```python
from build123d import *

# Parameters (mm, degrees)
SKETCH_1_R      = 40.9
SKETCH_1_R_2    = 1.55
EXTRUDE_1_DEPTH = 30


with BuildPart() as part:
    # 草图1 → 凸台-拉伸1 (new body)
    with BuildSketch(Plane(origin=(0, 0, 0), x_dir=(1, 0, 0), z_dir=(0, 1, 0))):
        with BuildLine():
            ThreePointArc((2.968149583, 44.335990888), (0, 46.9), (-2.968149583, 44.335990888))
            ThreePointArc((-2.968149583, 44.335990888), (-3.557987573, 43.187596963), (-4.726563367, 42.638827361))
            ThreePointArc((-4.726563367, 42.638827361), (-9.998714121, 41.718529647), (-15.115253688, 40.148961455))
            ThreePointArc((-15.115253688, 40.148961455), (-16.405630214, 40.108391944), (-17.451956512, 40.864645036))
            ThreePointArc((-17.451956512, 40.864645036), (-21.259908884, 41.80462025), (-22.74331541, 38.173703045))
            ThreePointArc((-22.74331541, 38.173703045), (-22.748500974, 36.882699338), (-23.541359728, 35.863831114))
            ThreePointArc((-23.541359728, 35.863831114), (-36.569613773, 22.429296657), (-42.638827361, 4.726563367))
            ThreePointArc((-42.638827361, 4.726563367), (-43.187596963, 3.557987573), (-44.335990888, 2.968149583))
            ThreePointArc((-44.335990888, 2.968149583), (-46.9, 0), (-44.335990888, -2.968149583))
            ThreePointArc((-44.335990888, -2.968149583), (-43.187596963, -3.557987573), (-42.638827361, -4.726563367))
            ThreePointArc((-42.638827361, -4.726563367), (-30.334880913, -30.334880913), (-4.726563367, -42.638827361))
            ThreePointArc((-4.726563367, -42.638827361), (-3.557987573, -43.187596963), (-2.968149583, -44.335990888))
            ThreePointArc((-2.968149583, -44.335990888), (0, -46.9), (2.968149583, -44.335990888))
            ThreePointArc((2.968149583, -44.335990888), (3.557987573, -43.187596963), (4.726563367, -42.638827361))
            ThreePointArc((4.726563367, -42.638827361), (30.334880913, -30.334880913), (42.638827361, -4.726563367))
            ThreePointArc((42.638827361, -4.726563367), (43.187596963, -3.557987573), (44.335990888, -2.968149583))
            ThreePointArc((44.335990888, -2.968149583), (46.9, 0), (44.335990888, 2.968149583))
            ThreePointArc((44.335990888, 2.968149583), (43.187596963, 3.557987573), (42.638827361, 4.726563367))
            ThreePointArc((42.638827361, 4.726563367), (30.334880913, 30.334880913), (4.726563367, 42.638827361))
            ThreePointArc((4.726563367, 42.638827361), (3.557987573, 43.187596963), (2.968149583, 44.335990888))
        make_face()
        Circle(SKETCH_1_R, mode=Mode.SUBTRACT)
        with Locations((0, 43.9)):
            Circle(SKETCH_1_R_2, mode=Mode.SUBTRACT)
        with Locations((43.9, 0)):
            Circle(SKETCH_1_R_2, mode=Mode.SUBTRACT)
        with Locations((0, -43.9)):
            Circle(SKETCH_1_R_2, mode=Mode.SUBTRACT)
        with Locations((-43.9, 0)):
            Circle(SKETCH_1_R_2, mode=Mode.SUBTRACT)
        with Locations((-19.9, 39.130550724)):
            Circle(SKETCH_1_R_2, mode=Mode.SUBTRACT)
    extrude(amount=EXTRUDE_1_DEPTH)


solid = part.part
```
Part model, mm, in its own coordinate system. A direction names the side the tool comes from. Give positions to 0.01 mm unless a question says otherwise; leave off trailing zeros. Write each loop counter-clockwise with the first axis right and the second up, starting at its lowest first coordinate (ties: lowest second). Pieces come first, ordered by that corner, then holes. Notation, with made-up numbers: (1.25, 14) -> (39.25, 14) arc R24 cw to (39.25, 52) -> close; hole circle Ø2 at (70.25, 55). An arc over 180 degrees is marked (long way). Put each result on its own line as item: value. Start each with the question number.
Item 1: Which spindle directions (+Z, -Z, +X, -X, +Y, -Y) get a long thin tool onto all of the face, cutting with end or side? Do faces 1 (the face through (28, 30, 31)), 2 (the face through (-9.926, 14.79, -41.736)). Say none if no direction does.
Item 2: Cut at B-B (z = 0). List the corners of the cut face in (x, y).
Item 3: Cut at C-C (y = 19). List the corners of the cut face in (x, z), then the cut area to 3 significant figures.
Item 4: Wall check: L1, parallel to Z at x = 0, y = 16.5; L2, parallel to X at y = 3, z = 5.5. Give the ranges that are in metal, low to high. Write a range as [from, to].
Item 5: Cut at D-D (z = 24.5). List the corners of the cut face in (x, y).
Item 6: Pull direction Z, two halves, no side cores. Call faces 3 (the face through (0.1, 14.8, -46.9)), 4 (the face through (-42.422, 14.79, -0.466)), 5 (the face through (46.9, 14.8, 0.1)), 6 (the face through (-0.1, 14.8, 46.9)): pulls with the +Z half, pulls with the -Z half, needs draft (parallel to the pull), parting line crosses it, or undercut.
Item 7: Pin check, flat tips, straight feed: pin 1 Ø5 at (y, z) = (15, 37) entering from +X; pin 2 Ø12 at (y, z) = (6.5, -3.5) entering from -X; pin 3 Ø6 at (y, z) = (3.5, -36.5) entering from -X; pin 4 Ø1.5 at (x, y) = (8, 24.5) entering from -Z. Stop position of each tip, or through.
Item 8: Cut at A-A (x = 0). List the corners of the cut face in (y, z), then the cut area to 3 significant figures.
Answer list:
1. face 1: +Z, -Z, +X, -X, +Y
1. face 2: -Z, +Y, -Y
2. outline: (-46.9, 0) -> (-45.45, 0) -> (-45.45, 30) -> (-46.9, 30) -> close; (-42.35, 0) -> (-40.9, 0) -> (-40.9, 30) -> (-42.35, 30) -> close; (40.9, 0) -> (42.35, 0) -> (42.35, 30) -> (40.9, 30) -> close; (45.45, 0) -> (46.9, 0) -> (46.9, 30) -> (45.45, 30) -> close
3. outline: (-44.34, -2.97) arc R2 cw to (-42.64, -4.73) arc R42.9 ccw to (-23.54, -35.86) arc R2 cw to (-22.74, -38.17) arc R3 ccw to (-17.45, -40.86) arc R2 cw to (-15.12, -40.15) arc R42.9 ccw to (-4.73, -42.64) arc R2 cw to (-2.97, -44.34) arc R3 ccw to (2.97, -44.34) arc R2 cw to (4.73, -42.64) arc R42.9 ccw to (42.64, -4.73) arc R2 cw to (44.34, -2.97) arc R3 ccw to (44.34, 2.97) arc R2 cw to (42.64, 4.73) arc R42.9 ccw to (4.73, 42.64) arc R2 cw to (2.97, 44.34) arc R3 ccw to (-2.97, 44.34) arc R2 cw to (-4.73, 42.64) arc R42.9 ccw to (-42.64, 4.73) arc R2 cw to (-44.34, 2.97) arc R3 ccw to start; hole circle Ø3.1 at (-43.9, 0); hole circle Ø81.8 at (0, 0); hole circle Ø3.1 at (-19.9, -39.13); hole circle Ø3.1 at (0, -43.9); hole circle Ø3.1 at (0, 43.9); hole circle Ø3.1 at (43.9, 0)
3. area: 597 mm2
4. L1: z = [-46.9, -45.45], [-42.35, -40.9], [40.9, 42.35], [45.45, 46.9]
4. L2: x = [-42.55, -40.53], [40.53, 42.55]
5. outline: (-35.22, 0) -> (-32.75, 0) -> (-32.75, 30) -> (-35.22, 30) -> close; (32.75, 0) -> (35.22, 0) -> (35.22, 30) -> (32.75, 30) -> close
6. face 3: pulls with the -Z half
6. face 4: undercut
6. face 5: parting line crosses it
6. face 6: pulls with the +Z half
7. pin 1: stops at x = 25.5
7. pin 2: stops at x = -46.9
7. pin 3: stops at x = -26.8
7. pin 4: stops at z = -42.28
8. outline: (0, -46.9) -> (30, -46.9) -> (30, -45.45) -> (0, -45.45) -> close; (0, -42.35) -> (30, -42.35) -> (30, -40.9) -> (0, -40.9) -> close; (0, 40.9) -> (30, 40.9) -> (30, 42.35) -> (0, 42.35) -> close; (0, 45.45) -> (30, 45.45) -> (30, 46.9) -> (0, 46.9) -> close
8. area: 174 mm2
